```python
from build123d import *

# Parameters (mm, degrees)
SKETCH1_W                   = 12
SKETCH1_H                   = 60
BOSS_EXTRUDE1_DEPTH         = 81.375
TAP_DRILL_FOR_M5X0_8_TAP1_D = 4.2
FILLET1_R                   = 2


with BuildPart() as part:
    # Sketch1 → Boss-Extrude1 (new body)
    with BuildSketch(Plane(origin=(0, 0, 0), x_dir=(1, 0, 0), z_dir=(0, 1, 0))):
        Rectangle(SKETCH1_W, SKETCH1_H)
    extrude(amount=-BOSS_EXTRUDE1_DEPTH)

    # Tap Drill for M5x0.8 Tap1 (through all)
    with Locations(Plane(origin=(0, 0, -10), x_dir=(0, 0, 1), z_dir=(0, 1, 0))):
        with Locations((0, 0), (20, 0), (-15, 0), (35, 0)):
            Hole(TAP_DRILL_FOR_M5X0_8_TAP1_D / 2)

    # Fillet1
    fillet1_edges = [part.edges().sort_by_distance(p)[0] for p in [
        (-6, -40.6875, -30),
        (-6, -40.6875, 30),
        (6, -40.6875, 30),
        (6, -40.6875, -30),
    ]]
    fillet(fillet1_edges, radius=FILLET1_R)


solid = part.part
```
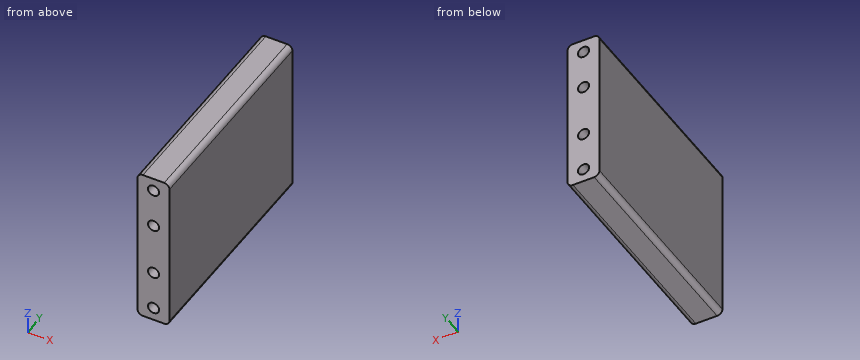
The model under review builds one solid part; all positions refer to its coordinate system, in mm. Give positions to 0.01 mm unless a question says otherwise; leave off trailing zeros. Write each loop counter-clockwise with the first axis right and the second up, starting at its lowest first coordinate (ties: lowest second). Pieces come first, ordered by that corner, then holes. Notation, with made-up numbers: (39.5, -11) -> (78.5, -11) arc R15 cw to (78.5, 13) -> close; hole circle Ø9 at (-32, 72). An arc over 180 degrees is marked (long way). Answer in a Markdown table with one row per item.
1) Clearance check with flat-ended pins moving along their axes: P1, Ø4, axis at x = 0, z = 25, coming from the -Y side; P2, Ø5, axis at x = 0, z = -25, coming from the +Y side. State where each tip first meets the part, or that it passes through.
Worked answers:
| item | result |
|---|---|
| P1 | through |
| P2 | y = 0 |
2) Add section C-C on x = 0. State the section outline as (y, z) points (3 decimals), plus the area to 3 significant figures.
Worked answers:
| item | result |
|---|---|
| outline | (-81.375, -30) -> (0, -30) -> (0, -27.1) -> (-81.375, -27.1) -> close; (-81.375, -22.9) -> (0, -22.9) -> (0, -12.1) -> (-81.375, -12.1) -> close; (-81.375, -7.9) -> (0, -7.9) -> (0, 7.9) -> (-81.375, 7.9) -> close; (-81.375, 12.1) -> (0, 12.1) -> (0, 22.9) -> (-81.375, 22.9) -> close; (-81.375, 27.1) -> (0, 27.1) -> (0, 30) -> (-81.375, 30) -> close |
| area | 3,520 mm² |
3) Add section B-B on z = 25. State the section outline as (x, y) points (3 decimals).
Worked answers:
| item | result |
|---|---|
| outline | (-6, -81.375) -> (-2.1, -81.375) -> (-2.1, 0) -> (-6, 0) -> close; (2.1, -81.375) -> (6, -81.375) -> (6, 0) -> (2.1, 0) -> close |
4) Add section A-A on y = -33. State the section outline as (x, z) points, plus the area to 3 significant figures.
Worked answers:
| item | result |
|---|---|
| outline | (-6, -28) arc R2 ccw to (-4, -30) -> (4, -30) arc R2 ccw to (6, -28) -> (6, 28) arc R2 ccw to (4, 30) -> (-4, 30) arc R2 ccw to (-6, 28) -> close; hole circle Ø4.2 at (0, -25); hole circle Ø4.2 at (0, -10); hole circle Ø4.2 at (0, 10); hole circle Ø4.2 at (0, 25) |
| area | 661 mm² |
5) For L1, parallel to Z at x = -0.25, y = -59; L2, parallel to Z at x = 1.75, y = -17.5; L3, parallel to X at y = -28.5, z = 10, list the stretches that pass through material, from the lowest coordinate up. Write a range as [from, to].
Worked answers:
| item | result |
|---|---|
| L1 | [-30, -27.09], [-22.91, -12.09], [-7.91, 7.91], [12.09, 22.91], [27.09, 30] |
| L2 | [-30, -26.16], [-23.84, -11.16], [-8.84, 8.84], [11.16, 23.84], [26.16, 30] |
| L3 | [-6, -2.1], [2.1, 6] |
